Model file for the job. Use its own axes, mm. A direction names the side the tool comes from. Coordinates: 2 decimals unless noted, no trailing zeros. Order: outer loops, then holes, each group sorted by start corner. A loop starts at its lowest first (then second) coordinate and runs counter-clockwise, first axis right, second up.
from build123d import *

# Parameters (mm, degrees)
BOSS_EXTRUDE2_DEPTH = 19.05
SKETCH3_R           = 3.175
CUT_EXTRUDE1_DEPTH  = 19.05
SKETCH4_R           = 3.175
CUT_EXTRUDE2_DEPTH  = 19.05


with BuildPart() as part:
    # Sketch2 → Boss-Extrude2 (new body)
    with BuildSketch(Plane.XY):
        Polygon((0, 0), (0, 25.4), (2.54, 25.4), (2.54, 2.54), (19.05, 2.54), (19.05, 0), align=None)
    extrude(amount=BOSS_EXTRUDE2_DEPTH)

    # Sketch3 → Cut-Extrude1 (cut)
    with BuildSketch(Plane(origin=(2.54, 0, 0), x_dir=(0, 0, -1), z_dir=(1, 0, 0))):
        with Locations((-9.525, 15.24)):
            Circle(SKETCH3_R)
    extrude(amount=-CUT_EXTRUDE1_DEPTH, mode=Mode.SUBTRACT)

    # Sketch4 → Cut-Extrude2 (cut)
    with BuildSketch(Plane(origin=(0, 2.54, 0), x_dir=(1, 0, 0), z_dir=(0, 1, 0))):
        with Locations((11.334166685, -9.525)):
            Circle(SKETCH4_R)
    extrude(amount=-CUT_EXTRUDE2_DEPTH, mode=Mode.SUBTRACT)


solid = part.part
Q1. Drop flat-ended pins along their axis: P1, Ø3, axis at x = 9.5, z = 7, coming from the -Y side; P2, Ø9.5, axis at y = 13.5, z = 6, coming from the +X side. Give the stop position or say it passes through.
Established:
P1: stops at y = 0
P2: stops at x = 2.54
Q2. Mould opens along X. For faces 3 (the face through (8.162, 1.288, 9.385)), 4 (the face through (19.05, 1, 9)), 5 (the face through (1.29, 12.14, 10.21)) say: pulls with the +X half, pulls with the -X half, needs draft (parallel to the pull), parting line crosses it, or undercut.
Established:
face 3: undercut
face 4: pulls with the +X half
face 5: needs draft
Q3. Cut at D-D, the plane x = 8.75. List the corners of the cut face in (y, z).
Established:
outline: (0, 0) - (2.54, 0) - (2.54, 7.68) - (0, 7.68) - close; (0, 11.37) - (2.54, 11.37) - (2.54, 19.05) - (0, 19.05) - close
Q4. Probe line 1 (Y direction, x = 15, z = 4); line 2 (X direction, y = 1.75, z = 11.75). List the from-to ranges inside material, lowest first.
Established:
line 1: y = 0 to 2.54
line 2: x = 0 to 9.07, 13.6 to 19.05
Q5. Cut at B-B, the plane x = 1.5. List the corners of the cut face in (y, z) (3 decimals).
Established:
outline: (0, 0) - (25.4, 0) - (25.4, 19.05) - (0, 19.05) - close; hole circle Ø6.35 at (15.24, 9.525)
Q6. Which spindle directions (+Z, -Z, +X, -X, +Y, -Y) get a long thin tool onto all of the face, cutting with end or side? Do faces 1 (the face through (9, 2.54, 12)), 2 (the face through (1, 25.4, 9)). Say none if no direction does.
Established:
face 1: +Z, -Z, +X, +Y
face 2: +Z, -Z, +X, -X, +Y
Q7. Cut at C-C, the plane z = 8.25. List the corners of the cut face in (x, y), plus the area to 3 significant figures.
Established:
outline: (0, 0) - (8.43, 0) - (8.43, 2.54) - (2.54, 2.54) - (2.54, 12.33) - (0, 12.33) - close; (0, 18.15) - (2.54, 18.15) - (2.54, 25.4) - (0, 25.4) - close; (14.24, 0) - (19.05, 0) - (19.05, 2.54) - (14.24, 2.54) - close
area: 76.9 mm2
Q8. Cut at A-A, the plane y = 15.24. List the corners of the cut face in (x, z).
Established:
outline: (0, 0) - (2.54, 0) - (2.54, 6.35) - (0, 6.35) - close; (0, 12.7) - (2.54, 12.7) - (2.54, 19.05) - (0, 19.05) - close
